from build123d import *

# Parameters (mm, degrees)
SKETCH2_W           = 56
SKETCH2_H           = 40
SKETCH2_W_2         = 40
SKETCH2_H_2         = 28.571428572
BOSS_EXTRUDE2_DEPTH = 3
SKETCH3_R           = 1.5
CUT_EXTRUDE1_DEPTH  = 4
FILLET1_R           = 2


with BuildPart() as part:
    # Sketch2 → Boss-Extrude2 (new body)
    with BuildSketch(Plane(origin=(0, 0, 0), x_dir=(1, 0, 0), z_dir=(0, 1, 0))):
        Rectangle(SKETCH2_W, SKETCH2_H)
        Rectangle(SKETCH2_W_2, SKETCH2_H_2, mode=Mode.SUBTRACT)
    extrude(amount=BOSS_EXTRUDE2_DEPTH)

    # Sketch3 → Cut-Extrude1 (cut, through all)
    with BuildSketch(Plane(origin=(0, 0, 0), x_dir=(-1, 0, 0), z_dir=(0, -1, 0))):
        with Locations((24, -16)):
            Circle(SKETCH3_R)
        with Locations((-24, 16)):
            Circle(SKETCH3_R)
        with Locations((-24, -16)):
            Circle(SKETCH3_R)
        with Locations((24, 16)):
            Circle(SKETCH3_R)
    extrude(amount=-CUT_EXTRUDE1_DEPTH, mode=Mode.SUBTRACT)

    # Fillet1
    fillet1_edges = [part.edges().sort_by_distance(p)[0] for p in [
        (28, 1.5, 20),
        (-28, 1.5, 20),
        (-28, 1.5, -20),
        (28, 1.5, -20),
    ]]
    fillet(fillet1_edges, radius=FILLET1_R)


solid = part.part
Here's how the part is built. I have some questions about the finished solid (model axes, mm). A direction names the side the tool comes from. Round coordinates to 2 decimals unless told otherwise and drop trailing zeros. Write each loop counter-clockwise with the first axis right and the second up, starting at its lowest first coordinate (ties: lowest second). Pieces come first, ordered by that corner, then holes.
1. I need wall thicknesses on L1, parallel to Z at x = 24, y = 2.4; L2, parallel to X at y = 1.4, z = -2.5; L3, parallel to Z at x = 1, y = 1.55. Which ranges of each line are inside material? Lowest first, please.
2. Suppose I cut it at A-A (z = -16). List the corners of the cut face in (x, y) for me.
3. Suppose I cut it at C-C (y = 2). List the corners of the cut face in (x, z) for me, and give its area (3 significant figures).
4. If we mould it in two halves opening along X, with no side actions, what happens to faces 3 (the cylindrical face through (-27.43, 1.52, -19.4)), 4 (the cylindrical face through (25.5, 1.48, 15.93)), 5 (the flat face through (28, 1, 0))? For each: released by +X, released by -X, zero draft, split by the parting line, or undercut.
5. Suppose I cut it at B-B (x = 1). List the corners of the cut face in (y, z) for me, and give its area (3 significant figures).
6. Suppose I cut it at D-D (z = 12). List the corners of the cut face in (x, y) for me.
7. For faces 1 (the flat face through (0, 1, 14.286)), 2 (the flat face through (0, 1, 20)), which set-ups out of +Z, -Z, +X, -X, +Y, -Y let a thin tool reach every point of the face, with its end or its side?
Answer sheet:
1. L1: z = -20 to -17.5, -14.5 to 14.5, 17.5 to 20
1. L2: x = -28 to -20, 20 to 28
1. L3: z = -20 to -14.29, 14.29 to 20
2. outline: (-28, 0) - (-25.5, 0) - (-25.5, 3) - (-28, 3) - close; (-22.5, 0) - (22.5, 0) - (22.5, 3) - (-22.5, 3) - close; (25.5, 0) - (28, 0) - (28, 3) - (25.5, 3) - close
3. outline: (-28, -18) arc R2 ccw to (-26, -20) - (26, -20) arc R2 ccw to (28, -18) - (28, 18) arc R2 ccw to (26, 20) - (-26, 20) arc R2 ccw to (-28, 18) - close; hole circle Ø3 at (-24, -16); hole circle Ø3 at (-24, 16); hole (-20, -14.29) - (20, -14.29) - (20, 14.29) - (-20, 14.29) - close; hole circle Ø3 at (24, -16); hole circle Ø3 at (24, 16)
3. area: 1,070 mm2
4. face 3: released by -X
4. face 4: undercut
4. face 5: released by +X
5. outline: (0, -20) - (3, -20) - (3, -14.29) - (0, -14.29) - close; (0, 14.29) - (3, 14.29) - (3, 20) - (0, 20) - close
5. area: 34.3 mm2
6. outline: (-28, 0) - (-20, 0) - (-20, 3) - (-28, 3) - close; (20, 0) - (28, 0) - (28, 3) - (20, 3) - close
7. face 1: +Y, -Y
7. face 2: +Z, +X, -X, +Y, -Y
